Check sheet for the modelled part. Datum: model origin and axes. Units: mm. Face numbers are marked on the shaded views. A direction names the side the tool comes from. Coordinates: 2 decimals unless noted, no trailing zeros. Loops run counter-clockwise (first coordinate to the right, second up) from the corner with the lowest first, then second, coordinate; pieces in that order, holes last.
```python
from build123d import *

# Parameters (mm, degrees)
SKETCH1_R           = 2.7
BOSS_EXTRUDE1_DEPTH = 2.7
CUT_EXTRUDE1_DEPTH  = 1
SKETCH3_R           = 1.5
BOSS_EXTRUDE2_DEPTH = 6


with BuildPart() as part:
    # Sketch1 → Boss-Extrude1 (new body)
    with BuildSketch(Plane(origin=(0, 0, 0), x_dir=(1, 0, 0), z_dir=(0, 1, 0))):
        Circle(SKETCH1_R)
    extrude(amount=BOSS_EXTRUDE1_DEPTH)

    # Sketch2 → Cut-Extrude1 (cut)
    with BuildSketch(Plane(origin=(0, 2.7, 0), x_dir=(1, 0, 0), z_dir=(0, 1, 0))):
        Polygon((0, 1.443375673), (-1.25, 0.721687836), (-1.25, -0.721687836), (0, -1.443375673), (1.25, -0.721687836), (1.25, 0.721687836), align=None)
    extrude(amount=-CUT_EXTRUDE1_DEPTH, mode=Mode.SUBTRACT)

    # Sketch3 → Boss-Extrude2 (add)
    with BuildSketch(Plane.XZ):
        Circle(SKETCH3_R)
    extrude(amount=BOSS_EXTRUDE2_DEPTH)


solid = part.part
```
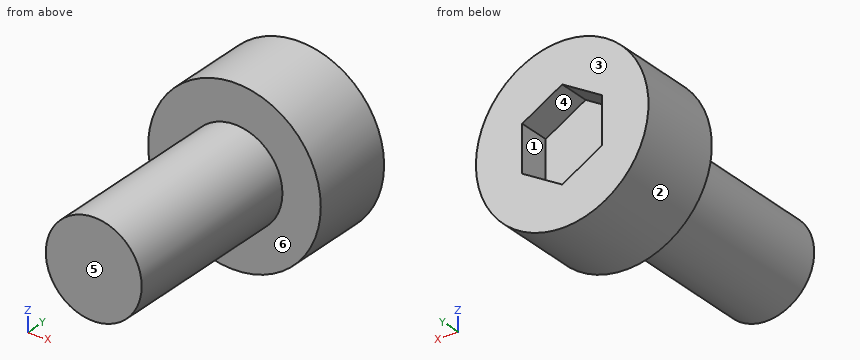
1) Depth check by flat-ended pin: pin 1 (0.8 mm diameter, centred on x = 0, z = -0.5, fed in from +Y). Enter the tip coordinate at first touch or a pass-through.
Answer sheet:
pin 1: stops at y = 1.7
2) Section check D-D on y = -0.25. Enter the section's corners in (x, z).
Answer sheet:
outline: circle Ø3 at (0, 0)
3) Scan lines: line 1 (Y direction, x = -1, z = 0.1); line 2 (Y direction, x = 1.45, z = 0.95); line 3 (Z direction, x = -0.95, y = -3). Record each from-to range of solid material in increasing order.
Answer sheet:
line 1: y = -6 to 1.7
line 2: y = 0 to 2.7
line 3: z = -1.16 to 1.16
4) Set-up check for the marked faces 4, 5 and 6: record each of +Z, -Z, +X, -X, +Y, -Y from which the full face is reachable in a straight line by a thin tool's end or side.
Answer sheet:
face 4: +Y
face 5: +Z, -Z, +X, -X, -Y
face 6: -Y
5) Mould release check, pull along X, two halves, no side actions. Record for the marked faces 1, 2 and 3: +X half, -X half, draft (parallel to the pull), parting line (faces both ways), or undercut.
Answer sheet:
face 1: undercut
face 2: parting line
face 3: draft
6) Section check A-A on z = 0. Enter the section's corners in (x, y).
Answer sheet:
outline: (-2.7, 0) - (-1.5, 0) - (-1.5, -6) - (1.5, -6) - (1.5, 0) - (2.7, 0) - (2.7, 2.7) - (1.25, 2.7) - (1.25, 1.7) - (-1.25, 1.7) - (-1.25, 2.7) - (-2.7, 2.7) - close
7) Section check C-C on x = -1.15. Enter the section's corners in (y, z).
Answer sheet:
outline: (-6, -0.96) - (0, -0.96) - (0, -2.44) - (2.7, -2.44) - (2.7, -0.78) - (1.7, -0.78) - (1.7, 0.78) - (2.7, 0.78) - (2.7, 2.44) - (0, 2.44) - (0, 0.96) - (-6, 0.96) - close
8) Section check B-B on y = 0.75. Enter the section's corners in (x, z), plus the area to 3 significant figures.
Answer sheet:
outline: circle Ø5.4 at (0, 0)
area: 22.9 mm2
